Verification items for the finished model (mm, model axes). A direction names the side the tool comes from. Coordinates: 2 decimals unless noted, no trailing zeros. Write each loop counter-clockwise with the first axis right and the second up, starting at its lowest first coordinate (ties: lowest second). Pieces come first, ordered by that corner, then holes. Notation, with made-up numbers: (8, 32) -> (36, 32) arc R30 ccw to (36, 60) -> close; hole circle Ø7 at (-4, -6.75). An arc over 180 degrees is marked (long way). Write item = value, one per line. Start each with the question number.
(1) Section check D-D (z = 527.5). Record the cut outline in (x, y) (3 decimals), plus the area to 3 significant figures.
(2) Section check B-B (x = 0). State how many separate pieces and enclosed holes the cut face has, plus the area to 3 significant figures.
(3) Mould release check, pull along X, two halves, no side actions. Record for faces 3 (the face through (25.4, 0, 307)), 4 (the face through (-4.29, -11.09, 74.52)), 5 (the face through (17, -12.7, 307)), 6 (the face through (15, 9.525, 307)): released by +X, released by -X, zero draft, split by the parting line, or undercut.
(4) Set-up check for faces 1 (the face through (-15, -9.525, 307)), 2 (the face through (0, 10, 12.7)): record each of +Z, -Z, +X, -X, +Y, -Y from which the full face is reachable in a straight line by a thin tool's end or side.
(5) Material ranges on probe 1 along Z at (x, y) = (0, 11.45); probe 2 along Y at (x, z) = (-17, 284.5) (3 decimals); probe 3 along X at (y, z) = (11.5, 534.15), recorded low to high. Write a range as [from, to].
(6) Section check A-A (z = 88.15). Record the cut outline in (x, y) (1 decimal).
(7) Section check C-C (z = 397). Record the cut outline in (x, y) (3 decimals).
Autodesk Inventor part; units mm, degrees
ref_plane "Start Plane" through (0, 0, 12.7) normal (0, 0, 1) x (1, 0, 0)
ref_plane "End Plane" through (0, 0, 609.6) normal (0, 0, 1) x (1, 0, 0)
ref_plane "Work Plane5" through (25.4, 498.475, 12.7) normal (0, 0, -1) x (-1, 0, 0)
ref_plane "Start Plane" through (0, 0, 12.7) normal (0, 0, 1) x (1, 0, 0)
ref_plane "End Plane" through (0, 0, 609.6) normal (0, 0, 1) x (1, 0, 0)
sketch "Sketch" plane through (0, 0, 0) normal (0, 0, 1) x (1, 0, 0)
  line L0 (-25.4, -12.7) -> (25.4, -12.7)
  line L1 (25.4, -12.7) -> (25.4, 12.7)
  line L2 (25.4, 12.7) -> (-25.4, 12.7)
  line L3 (-25.4, 12.7) -> (-25.4, -12.7)
  line L4 (-25.4, -12.7) -> (25.4, 12.7) construction
  line L5 (25.4, -12.7) -> (-25.4, 12.7) construction
  line L6 (-22.225, -9.525) -> (22.225, -9.525)
  line L7 (22.225, -9.525) -> (22.225, 9.525)
  line L8 (22.225, 9.525) -> (-22.225, 9.525)
  line L9 (-22.225, 9.525) -> (-22.225, -9.525)
  line L10 (-22.225, -9.525) -> (22.225, 9.525) construction
  line L11 (22.225, -9.525) -> (-22.225, 9.525) construction
  point P0 (0, 0)
  point P1 (0, 0)
  dimension "d0" = 50.8
  dimension "d1" = 25.4
  dimension "d2" = 3.175
  dimension "d3" = 3.175
extrude "Body" add sketch "Sketch" along normal up to surface (596.9 mm away) from surface at 12.7
sketch "Sketch4" plane through (0, 0, 0) normal (0, 0, 1) x (1, 0, 0)
  line L0 (0, 0) -> (10, 0)
ref_plane "Work Plane4" through (0, 0, 0) normal (0, -1, 0) x (1, 0, 0)
sketch "Sketch5" plane through (0, 0, 0) normal (0, -1, 0) x (1, 0, 0)
  line L0 (-2, 12.7) -> (12, 12.7)
  line L1 (-2, 609.6) -> (12, 609.6)
  dimension "d11" = 596.9
ref_plane "Work Plane5" through (25.4, 498.475, 12.7) normal (0, 0, -1) x (-1, 0, 0)
split "Split1" plane through (25.4, 498.475, 12.7) removes the side toward (0, 0, -1)
ref_plane "Work Plane6" through (25.4, -73.025, 609.6) normal (0, 0, 1) x (1, 0, 0)
split "Split2" plane through (25.4, -73.025, 609.6) removes the side toward (0, 0, 1)
sketch "Sketch6" plane through (-25.4, -12.7, 609.6) normal (0, -1, 0) x (1, 0, 0)
  line L0 (0, -203.2) -> (50.8, -203.2)
  line L1 (50.8, -393.7) -> (0, -393.7)
  line L2 (50.8, -596.9) -> (50.8, 0)
  line L3 (0, -596.9) -> (0, 0)
  point P0 (25.4, -298.45)
  point P1 (25.4, -75.45)
  point P2 (25.4, -521.45)
  dimension "d14" = 25.4
  dimension "d15" = 95.25
  dimension "d16" = 223
  dimension "d17" = 223
hole "Hole1" at (0, -12.7, 311.15) at (0, -12.7, 534.15) at (0, -12.7, 88.15) direction (0, 1, 0) diameter 28.575 end through all
equation "\"G_OFFSET_START\" = -12.7"
equation "\"G_OFFSET_END\" = -12.7"
equation "\"d6\" = -G_OFFSET_START"
equation "\"d7\" = length + G_OFFSET_END"
equation "\"G_L\" = d11"
properties part number "2x1inTubing"
Response:
q1.outline = (-25.4, -12.7) -> (-12.646, -12.7) -> (-12.646, -9.525) -> (-22.225, -9.525) -> (-22.225, 9.525) -> (-12.646, 9.525) -> (-12.646, 12.7) -> (-25.4, 12.7) -> close; (12.646, -12.7) -> (25.4, -12.7) -> (25.4, 12.7) -> (12.646, 12.7) -> (12.646, 9.525) -> (22.225, 9.525) -> (22.225, -9.525) -> (12.646, -9.525) -> close
q1.area = 283 mm2
q2.separate_pieces = 8
q2.enclosed_holes = 0
q2.area = 3,250 mm2
q3.face_3 = released by +X
q3.face_4 = undercut
q3.face_5 = zero draft
q3.face_6 = undercut
q4.face_1 = +Z, -Z
q4.face_2 = -Z, +X, -X, +Y, -Y
q5.probe_1 = [12.7, 73.86], [102.44, 296.86], [325.44, 519.86], [548.44, 609.6]
q5.probe_2 = [-12.7, -9.525], [9.525, 12.7]
q5.probe_3 = [-25.4, -14.29], [14.29, 25.4]
q6.outline = (-25.4, -12.7) -> (-14.3, -12.7) -> (-14.3, -9.5) -> (-22.2, -9.5) -> (-22.2, 9.5) -> (-14.3, 9.5) -> (-14.3, 12.7) -> (-25.4, 12.7) -> close; (14.3, -12.7) -> (25.4, -12.7) -> (25.4, 12.7) -> (14.3, 12.7) -> (14.3, 9.5) -> (22.2, 9.5) -> (22.2, -9.5) -> (14.3, -9.5) -> close
q7.outline = (-25.4, -12.7) -> (25.4, -12.7) -> (25.4, 12.7) -> (-25.4, 12.7) -> close; hole (-22.225, -9.525) -> (22.225, -9.525) -> (22.225, 9.525) -> (-22.225, 9.525) -> close
